Read the model definition and answer for the solid it produces. Units are mm, in the model's axes. Face numbers are marked on the shaded views. A direction names the side the tool comes from. Round coordinates to 2 decimals unless told otherwise and drop trailing zeros. Loops run counter-clockwise (first coordinate to the right, second up) from the corner with the lowest first, then second, coordinate; pieces in that order, holes last. Notation, with made-up numbers: (23.25, 77.25) -> (59.25, 77.25) arc R27 ccw to (59.25, 105.25) -> close; hole circle Ø2 at (-26.5, -6.5). An arc over 180 degrees is marked (long way). Put each result on its own line as item: value.
Autodesk Inventor part; units mm, degrees
ref_plane "YZ Plane" through (0, 0, 0) normal (1, 0, 0) x (0, 1, 0)
ref_plane "XZ Plane" through (0, 0, 0) normal (0, 1, 0) x (-1, 0, 0)
ref_plane "XY Plane" through (0, 0, 0) normal (0, 0, 1) x (1, 0, 0)
sketch "Эскиз1" plane through (0, 0, 0) normal (0, 0, 1) x (1, 0, 0)
  line L0 (0, 0) -> (0, 10)
  line L1 (0, 10) -> (50, 10)
  line L2 (50, 10) -> (50, 25)
  line L3 (50, 25) -> (70, 25)
  line L4 (70, 25) -> (70, 3)
  line L5 (0, 0) -> (4.3397, 0)
  line L6 (0, -10) -> (50, -10)
  line L7 (50, -10) -> (50, -25)
  line L8 (50, -25) -> (70, -25)
  line L9 (70, -25) -> (70, 3)
  line L10 (0, 10) -> (32, 10)
  line L11 (32, 10) -> (32, -10)
  dimension "d0" = 10
  dimension "d1" = 50
  dimension "d2" = 15
  dimension "d3" = 20
  dimension "d4" = 32
revolve "Вращение1" add sketch "Эскиз1" angle 360 about axis through (0, 0, 0) along (0, 1, 0)
fillet "Сопряжение1" radius 2 2 edges at (-50, 10, 0) (-50, -10, 0)
properties part number "Корпус сальника перегородка 1" material "Чугун, серый"
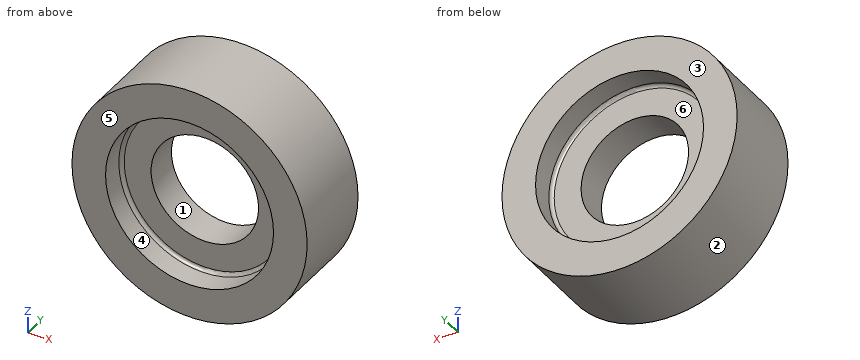
Item 1: Which of the six approach directions +Z, -Z, +X, -X, +Y, -Y give full straight-line access (tool end or side, diameter ignored) to the marked faces 4, 5 and 6?
Derived:
face 4: -Y
face 5: +Z, -Z, +X, -X, -Y
face 6: +Y
Item 2: The part is cut by section B-B (x = 0). Determine the outline of the cut face in (y, z).
Derived:
outline: (-25, -70) -> (25, -70) -> (25, -50) -> (12, -50) arc R2 cw to (10, -48) -> (10, -32) -> (-10, -32) -> (-10, -48) arc R2 cw to (-12, -50) -> (-25, -50) -> close; (-25, 50) -> (-12, 50) arc R2 cw to (-10, 48) -> (-10, 32) -> (10, 32) -> (10, 48) arc R2 cw to (12, 50) -> (25, 50) -> (25, 70) -> (-25, 70) -> close
Item 3: The part is cut by section A-A (z = 0). Determine the outline of the cut face in (x, y), then the cut area to 3 significant figures.
Derived:
outline: (-70, -25) -> (-50, -25) -> (-50, -12) arc R2 cw to (-48, -10) -> (-32, -10) -> (-32, 10) -> (-48, 10) arc R2 cw to (-50, 12) -> (-50, 25) -> (-70, 25) -> close; (32, -10) -> (48, -10) arc R2 cw to (50, -12) -> (50, -25) -> (70, -25) -> (70, 25) -> (50, 25) -> (50, 12) arc R2 cw to (48, 10) -> (32, 10) -> close
area: 2,720 mm^2
Item 4: For a pull along X with two mould halves and no side action, classify the marked faces 1, 2 and 3 as pulls with the +X half, pulls with the -X half, needs draft (parallel to the pull), parting line crosses it, or undercut.
Derived:
face 1: undercut
face 2: parting line crosses it
face 3: needs draft
Item 5: Flat-ended cylindrical pins translate along their axes: pin 1 Ø5 at (x, y) = (-36, 13.5) entering from +Z; pin 2 Ø3 at (x, z) = (-6, 35) entering from -Y; pin 3 Ø6 at (x, y) = (40.5, 3) entering from -Z. Find the tip coordinate at first contact, or state that the pin passes through.
Derived:
pin 1: stops at z = 61.46
pin 2: stops at y = -10
pin 3: stops at z = -59.11
Item 6: Find the intervals of material crossed by line 1 along Z through (x, y) = (0, -21); line 2 along Z through (x, y) = (0, 5.75), in increasing order.
Derived:
line 1: z = -70 to -50, 50 to 70
line 2: z = -70 to -32, 32 to 70
Item 7: The part is cut by section C-C (y = -21). Determine the outline of the cut face in (x, z).
Derived:
outline: circle Ø140 at (0, 0); hole circle Ø100 at (0, 0)
Item 8: The part is cut by section D-D (z = 61.5). Determine the outline of the cut face in (x, y), then the cut area to 3 significant figures.
Derived:
outline: (-33.43, -25) -> (33.43, -25) -> (33.43, 25) -> (-33.43, 25) -> close
area: 3,340 mm^2
